Work out the finished part from the listing and answer in its coordinate system (mm). Face numbers are marked on the shaded views. A direction names the side the tool comes from. Coordinates: 2 decimals unless noted, no trailing zeros. Loops run counter-clockwise (first coordinate to the right, second up) from the corner with the lowest first, then second, coordinate; pieces in that order, holes last. Notation, with made-up numbers: (-37.5, -5) - (21.5, -5) arc R10 cw to (21.5, 14) - close; hole circle Ø1 at (3.5, -9.5). An arc over 180 degrees is marked (long way). Write each question's results on one line, items separated by ' | '. Start each with the question number.
1. A cutting plane is placed at A-A on x = 14. Determine the outline of the cut face in (y, z), then the cut area to 3 significant figures.
2. Which of the six approach directions +Z, -Z, +X, -X, +Y, -Y give full straight-line access (tool end or side, diameter ignored) to the marked faces 1 and 2?
3. Determine the mould class of the marked faces 3 and 4 for opening direction X: released by +X, released by -X, zero draft, split by the parting line, or undercut.
4. A cutting plane is placed at D-D on x = 0. Determine the outline of the cut face in (y, z), then the cut area to 3 significant figures.
5. A cutting plane is placed at C-C on x = -48. Determine the outline of the cut face in (y, z).
6. Find the intervals of material crossed by line 1 along X through (y, z) = (1.65, 0); line 2 along Z through (x, y) = (-18, 0.5); line 3 along X through (y, z) = (-0.5, 9.5), in increasing order. Write a range as [from, to].
7. A cutting plane is placed at B-B on z = 0. Determine the outline of the cut face in (x, y).
from build123d import *

# Parameters (mm, degrees)
SKETCH_1_W          = 108
SKETCH_1_H          = 40
SKETCH_1_R          = 11.3
SKETCH_1_R_2        = 1.6
SKETCH_1_R_3        = 2.1
EXTRUDE_1_DEPTH     = 3
FILLET_1_R          = 1.5
CUT_EXTRUDE_1_DEPTH = 58.896459305
FILLET_2_R          = 3


with BuildPart() as part:
    # 草图1 → 凸台-拉伸1 (new, symmetric)
    with BuildSketch(Plane(origin=(0, 0, 0), x_dir=(1, 0, 0), z_dir=(0, 1, 0))):
        Rectangle(SKETCH_1_W, SKETCH_1_H)
        with Locations(Location((0, 0, 0), (0, 0, 270))):
            Circle(SKETCH_1_R, mode=Mode.SUBTRACT)
        with Locations(Location((0, 14, 0), (0, 0, 270))):
            Circle(SKETCH_1_R_2, mode=Mode.SUBTRACT)
        with Locations(Location((8, 13.856406461, 0), (0, 0, 270))):
            Circle(SKETCH_1_R_3, mode=Mode.SUBTRACT)
        with Locations(Location((8, -13.856406461, 0), (0, 0, 270))):
            Circle(SKETCH_1_R_3, mode=Mode.SUBTRACT)
        with Locations(Location((-8, -13.856406461, 0), (0, 0, 270))):
            Circle(SKETCH_1_R_3, mode=Mode.SUBTRACT)
        with Locations(Location((-8, 13.856406461, 0), (0, 0, 270))):
            Circle(SKETCH_1_R_3, mode=Mode.SUBTRACT)
        with Locations(Location((14, 0, 0), (0, 0, 270))):
            Circle(SKETCH_1_R_2, mode=Mode.SUBTRACT)
        with Locations(Location((0, -14, 0), (0, 0, 270))):
            Circle(SKETCH_1_R_2, mode=Mode.SUBTRACT)
        with Locations(Location((-14, 0, 0), (0, 0, 270))):
            Circle(SKETCH_1_R_2, mode=Mode.SUBTRACT)
        with Locations(Location((-48, -14, 0), (0, 0, 270))):
            Circle(SKETCH_1_R_3, mode=Mode.SUBTRACT)
        with Locations(Location((-48, 14, 0), (0, 0, 90))):
            Circle(SKETCH_1_R_3, mode=Mode.SUBTRACT)
        with Locations(Location((48, -14, 0), (0, 0, 90))):
            Circle(SKETCH_1_R_3, mode=Mode.SUBTRACT)
        with Locations(Location((48, 14, 0), (0, 0, 270))):
            Circle(SKETCH_1_R_3, mode=Mode.SUBTRACT)
    extrude(amount=EXTRUDE_1_DEPTH, both=True)

    # 圆角1
    fillet_1_edges = [part.edges().sort_by_distance(p)[0] for p in [
        (54, 0, 20),
        (-54, 0, 20),
        (-54, 0, -20),
        (54, 0, -20),
    ]]
    fillet(fillet_1_edges, radius=FILLET_1_R)

    # 草图3 → 切除-拉伸1 (cut, through all)
    with BuildSketch(Plane(origin=(0, 3, 0), x_dir=(1, 0, 0), z_dir=(0, 1, 0))):
        with BuildLine():
            Line((-39.153453709, 14), (-19.871537669, 2.263181541))
            ThreePointArc((-19.871537669, 2.263181541), (-18.057377806, 8.598319996), (-14.282856857, 14))
            Line((-14.282856857, 14), (-39.153453709, 14))
        make_face()
        Polygon((-43, 11.658623997), (-43, -11.658623997), (-23.846546291, 0), align=None)
        with BuildLine():
            Line((-39.153453709, -14), (-14.282856857, -14))
            ThreePointArc((-14.282856857, -14), (-18.057377806, -8.598319996), (-19.871537669, -2.263181541))
            Line((-19.871537669, -2.263181541), (-39.153453709, -14))
        make_face()
        with BuildLine():
            Line((14.282856857, -14), (39.153453709, -14))
            Line((39.153453709, -14), (19.871537669, -2.263181541))
            ThreePointArc((19.871537669, -2.263181541), (18.057377806, -8.598319996), (14.282856857, -14))
        make_face()
        Polygon((23.846546291, 0), (43, -11.658623997), (43, 11.658623997), align=None)
        with BuildLine():
            ThreePointArc((14.282856857, 14), (18.057377806, 8.598319996), (19.871537669, 2.263181541))
            Line((19.871537669, 2.263181541), (39.153453709, 14))
            Line((39.153453709, 14), (14.282856857, 14))
        make_face()
    extrude(amount=-CUT_EXTRUDE_1_DEPTH, mode=Mode.SUBTRACT)

    # 圆角2
    fillet_2_edges = [part.edges().sort_by_distance(p)[0] for p in [
        (-19.871537669, 0, 2.263181541),
        (-14.282856857, 0, 14),
        (-39.153453709, 0, 14),
        (-23.846546291, 0, 0),
        (-43, 0, 11.658623997),
        (-43, 0, -11.658623997),
        (23.846546291, 0, 0),
        (43, 0, -11.658623997),
        (43, 0, 11.658623997),
        (14.282856857, 0, 14),
        (19.871537669, 0, 2.263181541),
        (39.153453709, 0, 14),
        (19.871537669, 0, -2.263181541),
        (14.282856857, 0, -14),
        (39.153453709, 0, -14),
        (-14.282856857, 0, -14),
        (-19.871537669, 0, -2.263181541),
        (-39.153453709, 0, -14),
    ]]
    fillet(fillet_2_edges, radius=FILLET_2_R)


solid = part.part
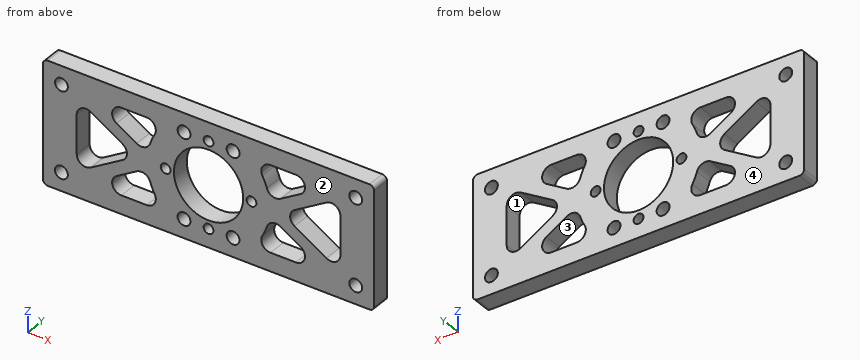
Values:
1) outline: (-3, -20) - (3, -20) - (3, -1.6) - (-3, -1.6) - close; (-3, 1.6) - (3, 1.6) - (3, 20) - (-3, 20) - close | area: 221 mm^2
2) face 1: +Y, -Y | face 2: +Z, -Z, +X, -X, -Y
3) face 3: undercut | face 4: zero draft
4) outline: (-3, -20) - (3, -20) - (3, -15.6) - (-3, -15.6) - close; (-3, -12.4) - (3, -12.4) - (3, -11.3) - (-3, -11.3) - close; (-3, 11.3) - (3, 11.3) - (3, 12.4) - (-3, 12.4) - close; (-3, 15.6) - (3, 15.6) - (3, 20) - (-3, 20) - close | area: 66.0 mm^2
5) outline: (-3, -20) - (3, -20) - (3, -16.1) - (-3, -16.1) - close; (-3, -11.9) - (3, -11.9) - (3, 11.9) - (-3, 11.9) - close; (-3, 16.1) - (3, 16.1) - (3, 20) - (-3, 20) - close
6) line 1: [-54, -43], [-26.62, -15.6], [-12.4, -11.3], [11.3, 12.4], [15.6, 26.62], [43, 54] | line 2: [-20, -13.04], [-8.72, 8.72], [13.04, 20] | line 3: [-54, -31.05], [-17.6, -6.12], [6.12, 17.6], [31.05, 54]
7) outline: (-54, -3) - (-43, -3) - (-43, 3) - (-54, 3) - close; (-26.62, -3) - (-15.6, -3) - (-15.6, 3) - (-26.62, 3) - close; (-12.4, -3) - (-11.3, -3) - (-11.3, 3) - (-12.4, 3) - close; (11.3, -3) - (12.4, -3) - (12.4, 3) - (11.3, 3) - close; (15.6, -3) - (26.62, -3) - (26.62, 3) - (15.6, 3) - close; (43, -3) - (54, -3) - (54, 3) - (43, 3) - close
